Autodesk Fusion 360 part; units mm, degrees
sketch "Skizze1" plane through (0, 0, 0) normal (0, 0, 1) x (1, 0, 0)
  line L0 (25, 25) -> (-25, 25)
  line L1 (-25, 25) -> (-25, -25)
  line L2 (-25, -25) -> (25, -25)
  line L3 (25, -25) -> (25, 25)
  line L4 (25, 25) -> (-25, -25) construction
  line L5 (-25, 25) -> (25, -25) construction
  line L6 (0, 25) -> (0, 21.5) construction
  circle A0 centre (0, 21.5) radius 2.5
  circle A1 centre (-21.5, 0) radius 2.5
  circle A2 centre (0, -21.5) radius 2.5
  circle A3 centre (21.5, 0) radius 2.5
  line L7 (-25, 25) -> (-19.6967, 19.6967)
  line L8 (25, 25) -> (19.6967, 19.6967)
  line L9 (25, -25) -> (19.6967, -19.6967)
  line L10 (-25, -25) -> (-19.6967, -19.6967)
  line L11 (0, 25) -> (0, 15) construction
  line L12 (25, 0) -> (15, 0) construction
  line L13 (0, -25) -> (0, -15) construction
  line L14 (-25, 0) -> (-15, 0) construction
  spline S0 degree 5 poles (0, -15) (1.2065, -15) (3.6254, -15.1465) (7.1572, -15.8132) (11.2047, -17.4413) (15.1309, -19.6326) (18.0012, -20.8352) (20.0511, -20.1301) (20.6752, -17.6735) (19.5115, -14.1604) (17.3962, -9.8731) (15.4021, -5.0946) (14.5897, -0.0184) (15.4512, 5.1337) (17.4986, 10.0731) (19.6685, 14.4705) (20.838, 17.9349) (20.126, 20.1337) (17.6793, 20.5662) (14.1665, 19.2783) (9.8729, 17.155) (5.088, 15.2723) (0.0153, 14.6011) (-5.1205, 15.5565) (-10.0405, 17.6249) (-14.4307, 19.7595) (-17.9076, 20.8718) (-20.1386, 20.1183) (-20.5833, 17.6619) (-19.2644, 14.1613) (-17.1004, 9.8864) (-15.2073, 5.1088) (-14.5882, 0.0204) (-15.6493, -5.152) (-17.8106, -10.1075) (-19.9406, -14.5038) (-20.9509, -17.9505) (-20.0386, -20.1219) (-17.7519, -20.5757) (-14.8416, -19.3727) (-11.0208, -17.3175) (-7.0919, -15.7983) (-3.6135, -15.1465) (-1.2065, -15) (0, -15) knots 0 0 0 0 0 0 0.025 0.05 0.075 0.1 0.125 0.15 0.175 0.2 0.225 0.25 0.275 0.3 0.325 0.35 0.375 0.4 0.425 0.45 0.475 0.5 0.525 0.55 0.575 0.6 0.625 0.65 0.675 0.7 0.725 0.75 0.775 0.8 0.825 0.85 0.875 0.9 0.925 0.95 0.975 1 1 1 1 1 1
  line L15 (-21.5565, -18.1362) -> (-17.8369, -21.2572)
  line L16 (-8.8743, -15) -> (8.8743, -15)
  line L17 (21.5565, 18.1362) -> (17.8369, 21.2572)
  line L18 (18.1362, -21.5565) -> (21.2572, -17.8369)
  line L19 (-18.1127, 21.5869) -> (-21.2807, 17.8065)
  line L20 (2.5, 19) -> (-2.5, 19)
  line L21 (-2.5, 19) -> (-2.5, 24)
  line L22 (-2.5, 24) -> (2.5, 24)
  line L23 (2.5, 24) -> (2.5, 19)
  line L24 (2.5, 19) -> (-2.5, 24) construction
  line L25 (-2.5, 19) -> (2.5, 24) construction
  line L26 (-19, 2.5) -> (-19, -2.5)
  line L27 (-24, 2.5) -> (-19, 2.5)
  line L28 (-24, -2.5) -> (-24, 2.5)
  line L29 (-19, -2.5) -> (-24, -2.5)
  line L30 (-2.5, -19) -> (2.5, -19)
  line L31 (-2.5, -24) -> (-2.5, -19)
  line L32 (2.5, -24) -> (-2.5, -24)
  line L33 (2.5, -19) -> (2.5, -24)
  line L34 (19, -2.5) -> (19, 2.5)
  line L35 (24, -2.5) -> (19, -2.5)
  line L36 (24, 2.5) -> (24, -2.5)
  line L37 (19, 2.5) -> (24, 2.5)
  point P0 (0, 21.5)
  dimension "d1" = 50
  dimension "d2" = 50
  dimension "d4" = 5
  dimension "d6" = 360
  dimension "d7" = 7.5
  dimension "d8" = 7.5
  dimension "d9" = 7.5
  dimension "d10" = 7.5
  dimension "d11" = 10
  dimension "d12" = 10
  dimension "d13" = 10
  dimension "d14" = 10
  dimension "d39" = 5
  dimension "d40" = 5
  dimension "d42" = 360
  dimension "d43" = 3.5
extrude "Extrusion1" add sketch "Skizze1" along normal blind 4 contours L0 L7 L8 S0 | L3 L8 L9 S0 | L1 L7 L10 S0 | L2 L9 L10 S0 | A0 | A0 L20 L23 | A0 L22 L23 | A0 L21 L22 | A0 L20 L21 | A1 | A1 L26 L29 | A1 L26 L27 | A1 L27 L28 | A1 L28 L29 | A2 | A2 L32 L33 | A2 L30 L33 | A2 L30 L31 | A2 L31 L32 | A3 | A3 L35 L36 | A3 L36 L37 | A3 L34 L37 | A3 L34 L35
sketch "Skizze9" plane through (0, 0, 4) normal (0, 0, 1) x (-1, 0, 0)
  spline S0 degree 5 poles (0, 15) (1.2065, 15) (3.6135, 15.1465) (7.0919, 15.7983) (11.0208, 17.3175) (14.8416, 19.3727) (17.7519, 20.5757) (20.0386, 20.1219) (20.9509, 17.9505) (19.9406, 14.5038) (17.8106, 10.1075) (15.6493, 5.152) (14.5882, -0.0204) (15.2073, -5.1088) (17.1004, -9.8864) (19.2644, -14.1613) (20.5833, -17.6619) (20.1386, -20.1183) (17.9076, -20.8718) (14.4307, -19.7595) (10.0405, -17.6249) (5.1205, -15.5565) (-0.0153, -14.6011) (-5.088, -15.2723) (-9.8729, -17.155) (-14.1665, -19.2783) (-17.6793, -20.5662) (-20.126, -20.1337) (-20.838, -17.9349) (-19.6685, -14.4705) (-17.4986, -10.0731) (-15.4512, -5.1337) (-14.5897, 0.0184) (-15.4021, 5.0946) (-17.3962, 9.8731) (-19.5115, 14.1604) (-20.6752, 17.6735) (-20.0511, 20.1301) (-18.0012, 20.8352) (-15.1309, 19.6326) (-11.2047, 17.4413) (-7.1572, 15.8132) (-3.6254, 15.1465) (-1.2065, 15) (0, 15) knots -1 -1 -1 -1 -1 -1 -0.975 -0.95 -0.925 -0.9 -0.875 -0.85 -0.825 -0.8 -0.775 -0.75 -0.725 -0.7 -0.675 -0.65 -0.625 -0.6 -0.575 -0.55 -0.525 -0.5 -0.475 -0.45 -0.425 -0.4 -0.375 -0.35 -0.325 -0.3 -0.275 -0.25 -0.225 -0.2 -0.175 -0.15 -0.125 -0.1 -0.075 -0.05 -0.025 0 0 0 0 0 0
  line L0 (-25, 25) -> (-25, -25)
  line L1 (-25, -25) -> (25, -25)
  line L2 (25, -25) -> (25, 25)
  line L3 (25, 25) -> (-25, 25)
  line L4 (24, 24) -> (-24, 24)
  line L5 (-24, 24) -> (-24, -24)
  line L6 (-24, -24) -> (24, -24)
  line L7 (24, -24) -> (24, 24)
  line L8 (0, -25) -> (-5, -25)
  line L9 (-5, -25) -> (-5, -24)
  line L10 (-5, -25) -> (-6, -25)
  line L11 (-6, -25) -> (-6, -24)
  line L12 (0, -25) -> (0, -24) construction
  line L13 (6, -25) -> (6, -24)
  line L14 (5, -25) -> (5, -24)
  line L15 (5, -24) -> (-5, -24)
  line L16 (-5, -24) -> (-5, -23)
  line L17 (-5, -23) -> (5, -23)
  line L18 (5, -23) -> (5, -24)
  line L19 (25, 6) -> (24, 6)
  line L20 (25, 5) -> (24, 5)
  line L21 (23, 5) -> (24, 5)
  line L22 (23, -5) -> (23, 5)
  line L23 (25, -5) -> (24, -5)
  line L24 (25, -6) -> (24, -6)
  line L25 (24, -5) -> (23, -5)
  line L26 (-6, 25) -> (-6, 24)
  line L27 (-5, 25) -> (-5, 24)
  line L28 (-5, 23) -> (-5, 24)
  line L29 (5, 23) -> (-5, 23)
  line L30 (5, 25) -> (5, 24)
  line L31 (6, 25) -> (6, 24)
  line L32 (5, 24) -> (5, 23)
  line L33 (-25, -6) -> (-24, -6)
  line L34 (-25, -5) -> (-24, -5)
  line L35 (-23, -5) -> (-24, -5)
  line L36 (-23, 5) -> (-23, -5)
  line L37 (-25, 5) -> (-24, 5)
  line L38 (-25, 6) -> (-24, 6)
  line L39 (-24, 5) -> (-23, 5)
  dimension "d65" = -1
  dimension "d66" = 5
  dimension "d67" = 1
  dimension "d70" = 0
  dimension "d71" = 0
  dimension "d72" = 10
  dimension "d73" = 1
  dimension "d75" = 360
extrude "Extrusion12" add sketch "Skizze9" along normal blind 3 contours L0 L3 L4 L5 L26 L38 | L0 L5 L34 L37 | L3 L4 L27 L30 | L5 L35 L36 L39 | L4 L28 L29 L32 | L0 L1 L5 L6 L11 L33 | L2 L3 L4 L7 L19 L31 | L1 L6 L8 L9 L14 L15 | L2 L7 L20 L23 | L6 L15 L16 L17 L18 | L7 L21 L22 L25 | L1 L2 L6 L7 L13 L24
extrude "Extrusion13" cut sketch "Skizze9" along normal blind 2 contours L5 L35 L36 L39 | L4 L28 L29 L32 | L6 L15 L16 L17 L18 | L7 L21 L22 L25
chamfer "Fase1" distance 1 angle 45 4 edges at (23, 0, 7) (0, -23, 7) (-23, 0, 7) (0, 23, 7)
extrude "Extrusion14" cut sketch "Skizze1" along normal blind 2.5 contours A0 | A0 L20 L23 | A0 L22 L23 | A0 L21 L22 | A0 L20 L21 | A1 | A1 L26 L29 | A1 L26 L27 | A1 L27 L28 | A1 L28 L29 | A2 | A2 L32 L33 | A2 L30 L33 | A2 L30 L31 | A2 L31 L32 | A3 | A3 L35 L36 | A3 L36 L37 | A3 L34 L37 | A3 L34 L35
Read the model definition and answer for the solid it produces. Units are mm, in the model's axes. A direction names the side the tool comes from. Round coordinates to 2 decimals unless told otherwise and drop trailing zeros. One line per question, with ' | ' between items. Start each with the question number.
1. Section A-A (z = 5.25) is taken. Give the number of separate pieces and of enclosed holes in the cut face, and give its area (3 significant figures).
2. Find the intervals of material crossed by probe 1 along Y at (x, z) = (8.5, 5.25); probe 2 along X at (y, z) = (22, 1.5), in increasing order. Write a range as [from, to].
3. Each of these flat-tipped pins is pushed along its axis until it touches: pin 1 (1.5 mm diameter, centred on x = 21, y = -0.5, fed in from -Z); pin 2 (12 mm diameter, centred on x = 0.5, y = 12.5, fed in from +Z). Where does it stop, or does it pass through?
4. For faces 3 (the face through (-2.5, -22, 1)), 4 (the face through (15, 24, 5)), 5 (the face through (24.7, 19.7, 7)), 6 (the face through (-5, 24.5, 5.5)), 7 (the face through (0, -24, 5)), determine the directions among +Z, -Z, +X, -X, +Y, -Y from which every point of the face is accessible in a straight line to the end or side of a thin tool.
5. For a pull along Y with two mould halves and no side action, classify faces 1 (the face through (5, 24.5, 5.5)), 2 (the face through (-24.5, 5, 5.5)) as +Y half, -Y half, draft (parallel to the pull), parting line (faces both ways), or undercut.
Filled in:
1) separate pieces: 8 | enclosed holes: 0 | area: 188 mm²
2) probe 1: [-25, -24], [24, 25] | probe 2: [-25, -2.5], [2.5, 25]
3) pin 1: z = 2.5 | pin 2: z = 4
4) face 3: -Z | face 4: +Z | face 5: +Z, +X, -X, +Y, -Y | face 6: +Z, +Y, -Y | face 7: none
5) face 1: draft | face 2: undercut
